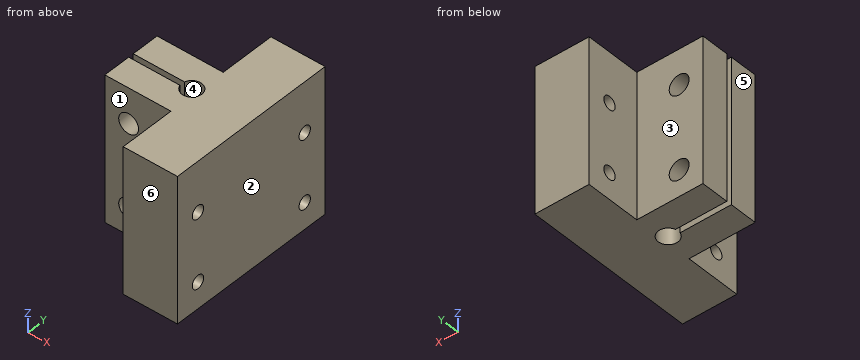
```python
from build123d import *

# Parameters (mm, degrees)
F1_DEPTH = 55
F2_R     = 2.5
F3_DEPTH = 45.501
F4_R     = 3.75
F5_DEPTH = 44.001


with BuildPart() as f1:
    # F0 (on Top) → F1 (new body)
    with BuildSketch(Plane.XY):
        with BuildLine():
            Line((63.350305, -26.724461), (63.350305, 38.275539))
            Line((63.350305, 38.275539), (42.850305, 38.275539))
            Line((42.850305, 38.275539), (42.850305, 17.275539))
            Line((42.850305, 17.275539), (17.850305, 17.275539))
            Line((17.850305, 17.275539), (17.850305, 6.775539))
            Line((17.850305, 6.775539), (37.236097, 6.775539))
            ThreePointArc((37.236097, 6.775539), (44.600305, 5.775539), (37.236097, 4.775539))
            Line((37.236097, 4.775539), (17.850305, 4.775539))
            Line((17.850305, 4.775539), (17.850305, -5.724461))
            Line((17.850305, -5.724461), (42.850305, -5.724461))
            Line((42.850305, -5.724461), (42.850305, -26.724461))
            Line((42.850305, -26.724461), (63.350305, -26.724461))
        make_face()
    extrude(amount=F1_DEPTH)

    # F2 (on face) → F3 (cut, through all)
    with BuildSketch(Plane.YZ.offset(63.350305)):
        with Locations((29.275539, 10)):
            Circle(F2_R)
        with Locations((29.275539, 36)):
            Circle(F2_R)
        with Locations((-17.724461, 10)):
            Circle(F2_R)
        with Locations((-17.724461, 36)):
            Circle(F2_R)
    extrude(amount=-F3_DEPTH, mode=Mode.SUBTRACT)

    # F4 (on face) → F5 (cut, through all)
    with BuildSketch(Plane.XZ.offset(5.724461)):
        with Locations((26.850305, 41.680109)):
            Circle(F4_R)
        with Locations((26.850305, 10)):
            Circle(F4_R)
    extrude(amount=-F5_DEPTH, mode=Mode.SUBTRACT)


solid = f1.part
```
Model file for the job. Use its own axes, mm. Face numbers are marked on the shaded views. A direction names the side the tool comes from. Give positions to 0.01 mm unless a question says otherwise; leave off trailing zeros. Loops run counter-clockwise (first coordinate to the right, second up) from the corner with the lowest first, then second, coordinate; pieces in that order, holes last. Notation, with made-up numbers: M -21.75,-17.5 L 4.25,-17.5 A19 cw 4.25,17.5 Z; hole C -14,40 d11. An arc over 180 degrees is marked long. Use one line per item in the form item = value.
Item 1: Slice it at A-A on z = 10. List the corners of the cut face in (x, y), and give its area (3 significant figures).
Filled in:
outline = M 17.85,-5.72 L 23.1,-5.72 L 23.1,4.78 L 17.85,4.78 Z; M 17.85,6.78 L 23.1,6.78 L 23.1,17.28 L 17.85,17.28 Z; M 30.6,-5.72 L 42.85,-5.72 L 42.85,-15.22 L 63.35,-15.22 L 63.35,26.78 L 42.85,26.78 L 42.85,17.28 L 30.6,17.28 L 30.6,6.78 L 37.24,6.78 A3.75 cw long 37.24,4.78 L 30.6,4.78 Z; M 42.85,-26.72 L 63.35,-26.72 L 63.35,-20.22 L 42.85,-20.22 Z; M 42.85,31.78 L 63.35,31.78 L 63.35,38.28 L 42.85,38.28 Z
area = 1,460 mm^2
Item 2: Slice it at D-D on x = 55.5. List the corners of the cut face in (y, z).
Filled in:
outline = M -26.72,0 L 38.28,0 L 38.28,55 L -26.72,55 Z; hole C -17.72,10 d5; hole C -17.72,36 d5; hole C 29.28,10 d5; hole C 29.28,36 d5
Item 3: Slice it at B-B on x = 32.5. List the corners of the cut face in (y, z).
Filled in:
outline = M -5.72,0 L 4.78,0 L 4.78,55 L -5.72,55 Z; M 6.78,0 L 17.28,0 L 17.28,55 L 6.78,55 Z
Item 4: Which spindle directions (+Z, -Z, +X, -X, +Y, -Y) get a long thin tool onto all of the face, cutting with end or side? Do the marked faces 1, 2 and 3. Say none if no direction does.
Filled in:
face_1 = +Z, -Z, -X, -Y
face_2 = +Z, -Z, +X, +Y, -Y
face_3 = +Z, -Z, -X, +Y
Item 5: Two-plate mould, pull along Y, no slides. Class the marked faces 4, 5 and 6: released by +Y, released by -Y, zero draft, split by the parting line, or undercut.
Filled in:
face_4 = undercut
face_5 = zero draft
face_6 = released by -Y
Item 6: Slice it at C-C on z = 36. List the corners of the cut face in (x, y), and give its area (3 significant figures).
Filled in:
outline = M 17.85,-5.72 L 42.85,-5.72 L 42.85,-15.22 L 63.35,-15.22 L 63.35,26.78 L 42.85,26.78 L 42.85,17.28 L 17.85,17.28 L 17.85,6.78 L 37.24,6.78 A3.75 cw long 37.24,4.78 L 17.85,4.78 Z; M 42.85,-26.72 L 63.35,-26.72 L 63.35,-20.22 L 42.85,-20.22 Z; M 42.85,31.78 L 63.35,31.78 L 63.35,38.28 L 42.85,38.28 Z
area = 1,620 mm^2
Item 7: Flat gauge pins, fed straight in: pin 1 Ø6 at (x, z) = (24.5, 27) entering from +Y; pin 2 Ø6 at (x, z) = (30, 33) entering from -Y; pin 3 Ø2 at (x, z) = (42.5, 15.5) entering from -Y; pin 4 Ø5 at (y, z) = (-13, 49) entering from -X. Where does each tip first touch, or does it go through?
Filled in:
pin_1 = 17.28
pin_2 = -5.72
pin_3 = -26.72
pin_4 = 42.85
Item 8: Drill centre lines: L1, parallel to Z at x = 50, y = 29; L2, parallel to Y at x = 28, z = 24.5; L3, parallel to Y at x = 60.5, z = 37. Where is each one in solid material? Low to high.
Filled in:
L1 = 0 to 7.52, 12.48 to 33.52, 38.48 to 55
L2 = -5.72 to 4.78, 6.78 to 17.28
L3 = -26.72 to -20.02, -15.43 to 26.98, 31.57 to 38.28
